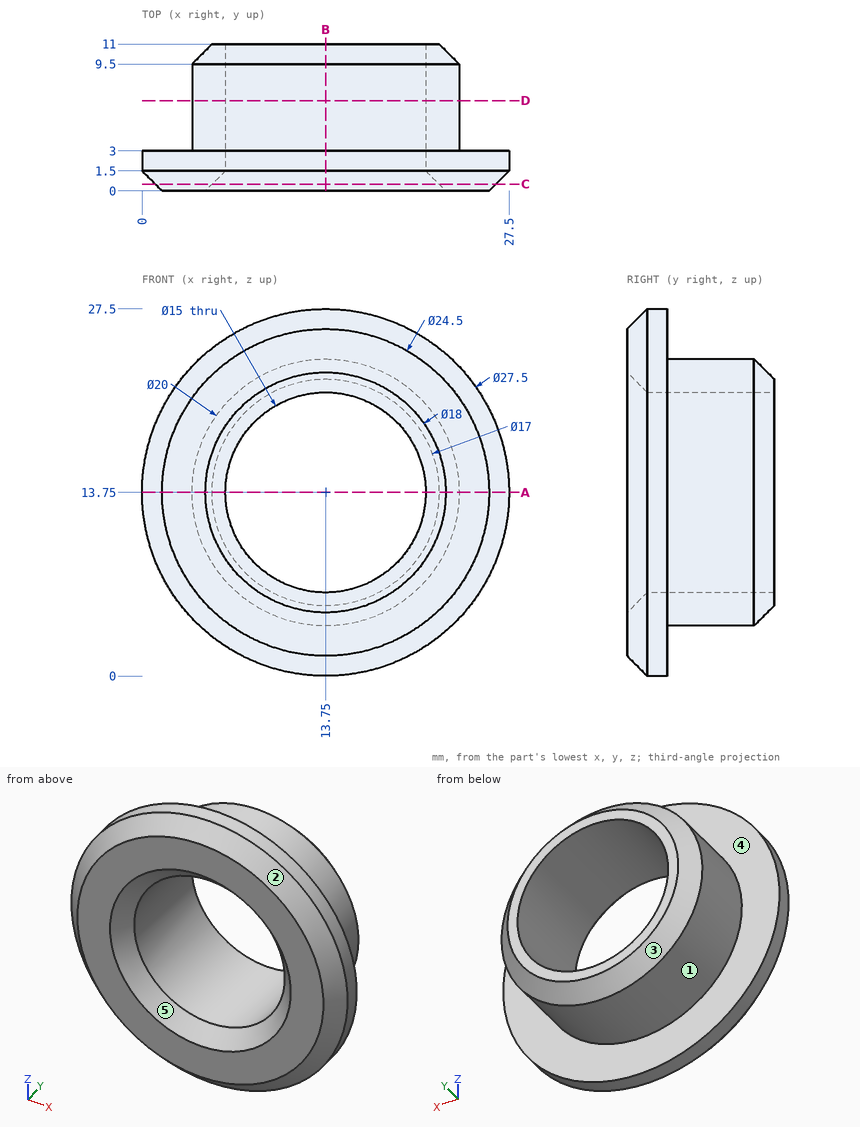
Print and shaded views of the part. All mm, measured from the part's lowest x, y and z. A direction names the side the tool comes from. Coordinates: 2 decimals unless noted, no trailing zeros. Loops run counter-clockwise (first coordinate to the right, second up) from the corner with the lowest first, then second, coordinate; pieces in that order, holes last. Notation, with made-up numbers: (59, 62) -> (92, 62) arc R9 cw to (92, 68) -> close; hole circle Ø4 at (34, 79.5). An arc over 180 degrees is marked (long way). Use a Markdown table: item, result. Add a question column.
Item 1: Probe probe 1 along X at (y, z) = (8.75, 13.75); probe 2 along Z at (x, y) = (19.75, 1.75); probe 3 along Y at (x, z) = (23.25, 8.25). List the from-to ranges inside material, lowest first.
Item 2: Band-saw the part on D-D on y = 6.75. Write the cut outline in (x, z), plus the area to 3 significant figures.
Item 3: Band-saw the part on B-B on x = 13.75. Write the cut outline in (y, z).
Item 4: Which spindle directions (+Z, -Z, +X, -X, +Y, -Y) get a long thin tool onto all of the face, cutting with end or side? Do the marked faces 1 and 2. Say none if no direction does.
Item 5: Pull direction X, two halves, no side cores. Call the marked faces 3, 4 and 5: +X half, -X half, draft (parallel to the pull), parting line (faces both ways), or undercut.
Item 6: Band-saw the part on A-A on z = 13.75. Write the cut outline in (x, y).
Item 7: Flat gauge pins, fed straight in: P1, Ø3, axis at x = 14, z = 21, coming from the +Y side; P2, Ø2, axis at x = 13.5, z = 6.5, coming from the -Y side; P3, Ø3, axis at x = 20.5, y = 6, coming from the -Z side. Where does each tip first touch, or does it go through?
Item 8: Band-saw the part on C-C on y = 0.5. Write the cut outline in (x, z), plus the area to 3 significant figures.
Geometry says:
| question | item | result |
|---|---|---|
| 1 | probe 1 | 3.75 to 6.25, 21.25 to 23.75 |
| 1 | probe 2 | 1.38 to 9.25, 18.25 to 26.12 |
| 1 | probe 3 | 0 to 3 |
| 2 | outline | circle Ø20 at (13.75, 13.75); hole circle Ø15 at (13.75, 13.75) |
| 2 | area | 137 mm² |
| 3 | outline | (0, 1.5) -> (1.5, 0) -> (3, 0) -> (3, 3.75) -> (9.5, 3.75) -> (11, 5.25) -> (11, 6.25) -> (1.5, 6.25) -> (0, 4.75) -> close; (0, 22.75) -> (1.5, 21.25) -> (11, 21.25) -> (11, 22.25) -> (9.5, 23.75) -> (3, 23.75) -> (3, 27.5) -> (1.5, 27.5) -> (0, 26) -> close |
| 4 | face 1 | +Y |
| 4 | face 2 | -Y |
| 5 | face 3 | parting line |
| 5 | face 4 | draft |
| 5 | face 5 | undercut |
| 6 | outline | (0, 1.5) -> (1.5, 0) -> (4.75, 0) -> (6.25, 1.5) -> (6.25, 11) -> (5.25, 11) -> (3.75, 9.5) -> (3.75, 3) -> (0, 3) -> close; (21.25, 1.5) -> (22.75, 0) -> (26, 0) -> (27.5, 1.5) -> (27.5, 3) -> (23.75, 3) -> (23.75, 9.5) -> (22.25, 11) -> (21.25, 11) -> close |
| 7 | P1 | y = 11 |
| 7 | P2 | y = 0.75 |
| 7 | P3 | z = 5.24 |
| 8 | outline | circle Ø25.5 at (13.75, 13.75); hole circle Ø17 at (13.75, 13.75) |
| 8 | area | 284 mm² |
